Geometry: see drawing. Coordinates: mm, zero at the bounding-box minimum. A direction names the side the tool comes from. Give positions to 0.01 mm unless a question says otherwise; leave off trailing zeros. Write each loop counter-clockwise with the first axis right and the second up, starting at its lowest first coordinate (ties: lowest second). Pieces come first, ordered by that corner, then holes. Notation, with made-up numbers: (-16.5, -26.5) -> (-5.5, -26.5) arc R17 cw to (-5.5, -11.5) -> close; hole circle Ø11 at (37.25, -1.75). An arc over 180 degrees is marked (long way). Use one line per item in the form item = value. Start each with the question number.
(1) Cut plane B-B, the plane x = 18.5. Output: boundary loops of the cut face in (y, z), and give its area (3 significant figures).
(2) Cut plane C-C, the plane y = 14. Output: boundary loops of the cut face in (x, z).
(3) Cut plane D-D, the plane y = 22. Output: boundary loops of the cut face in (x, z).
(4) Material intervals for line 1 along X through (y, z) = (13.5, 2.7); line 2 along Y through (x, z) = (18.5, 2.5); line 3 along X through (y, z) = (3.75, 1.05), sorted ascending. Write a range as from..to.
(5) Cut plane A-A, the plane z = 2.5. Output: boundary loops of the cut face in (x, y).
(6) First-contact query: P1, Ø5.5, axis at x = 18.5, y = 5, coming from the +Z side; P2, Ø1.5, axis at x = 9, z = 3, coming from the +Y side. Flat tips, straight axial feed; report the tip coordinate or a pass-through.
(7) Draft query along X for the marked faces 1, 2 and 3. Return one class per face: pulls with the +X half, pulls with the -X half, needs draft (parallel to the pull), parting line crosses it, or undercut.
(8) Set-up query: the marked faces 4, 5 and 6. Return all of +Z, -Z, +X, -X, +Y, -Y with unobstructed straight access to the full face (end or side cutting, diameter ignored); none if empty.
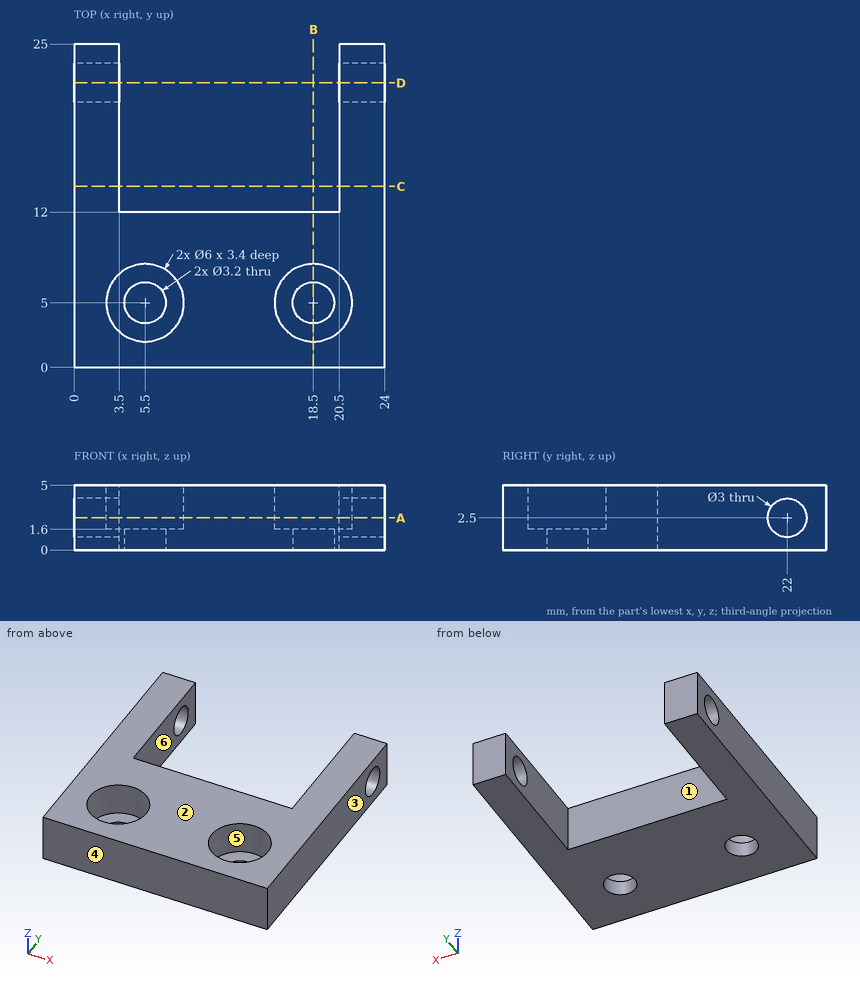
Geometry says:
q1.outline = (0, 0) -> (3.4, 0) -> (3.4, 1.6) -> (2, 1.6) -> (2, 5) -> (0, 5) -> close; (6.6, 0) -> (12, 0) -> (12, 5) -> (8, 5) -> (8, 1.6) -> (6.6, 1.6) -> close
q1.area = 34.5 mm^2
q2.outline = (0, 0) -> (3.5, 0) -> (3.5, 5) -> (0, 5) -> close; (20.5, 0) -> (24, 0) -> (24, 5) -> (20.5, 5) -> close
q3.outline = (0, 0) -> (3.5, 0) -> (3.5, 1) -> (0, 1) -> close; (0, 4) -> (3.5, 4) -> (3.5, 5) -> (0, 5) -> close; (20.5, 0) -> (24, 0) -> (24, 1) -> (20.5, 1) -> close; (20.5, 4) -> (24, 4) -> (24, 5) -> (20.5, 5) -> close
q4.line_1 = 0..3.5, 20.5..24
q4.line_2 = 0..2, 8..12
q4.line_3 = 0..4.5, 6.5..17.5, 19.5..24
q5.outline = (0, 0) -> (24, 0) -> (24, 20.5) -> (20.5, 20.5) -> (20.5, 12) -> (3.5, 12) -> (3.5, 20.5) -> (0, 20.5) -> close; (0, 23.5) -> (3.5, 23.5) -> (3.5, 25) -> (0, 25) -> close; (20.5, 23.5) -> (24, 23.5) -> (24, 25) -> (20.5, 25) -> close; hole circle Ø6 at (5.5, 5); hole circle Ø6 at (18.5, 5)
q6.P1 = 1.6
q6.P2 = 12
q7.face_1 = undercut
q7.face_2 = needs draft
q7.face_3 = pulls with the +X half
q8.face_4 = +Z, -Z, +X, -X, -Y
q8.face_5 = +Z
q8.face_6 = +Z, -Z, +Y
